Part print with two shaded views. Sizes in mm from the minimum x, y, z corner. Round coordinates to 2 decimals unless told otherwise and drop trailing zeros. Order: outer loops, then holes, each group sorted by start corner. A loop starts at its lowest first (then second) coordinate and runs counter-clockwise, first axis right, second up. Notation, with made-up numbers: (-15, 71.5) - (-2, 71.5) arc R18 cw to (-2, 85.5) - close; hole circle Ø10 at (0, -7.75). An arc over 180 degrees is marked (long way). Answer as CSV lines item,"result". Start each with the question number.
1. Pin check, flat tips, straight feed: pin 1 Ø8 at (x, z) = (75, 8) entering from +Y; pin 2 Ø3 at (x, z) = (85, 27.92) entering from +Y. Stop position of each tip, or through.
2. Pull direction Z, two halves, no side cores. Call the marked faces 1, 2 and 3: released by +Z, released by -Z, zero draft, split by the parting line, or undercut.
3. Band-saw the part on A-A on x = 65. List the corners of the cut face in (y, z) (3 decimals).
4. Band-saw the part on C-C on x = 85. List the corners of the cut face in (y, z) (3 decimals), then the cut area to 3 significant figures.
5. Band-saw the part on B-B on z = 19.5. List the corners of the cut face in (x, y), then the cut area to 3 significant figures.
6. Band-saw the part on D-D on x = 50. List the corners of the cut face in (y, z).
7. Wall check: line 1 along X through (y, z) = (6, 12); line 2 along Z through (x, y) = (15, 5.5); line 3 along Z through (x, y) = (75, 0.25) (3 decimals). Give the ranges that are in metal, low to high. Write a range as [from, to].
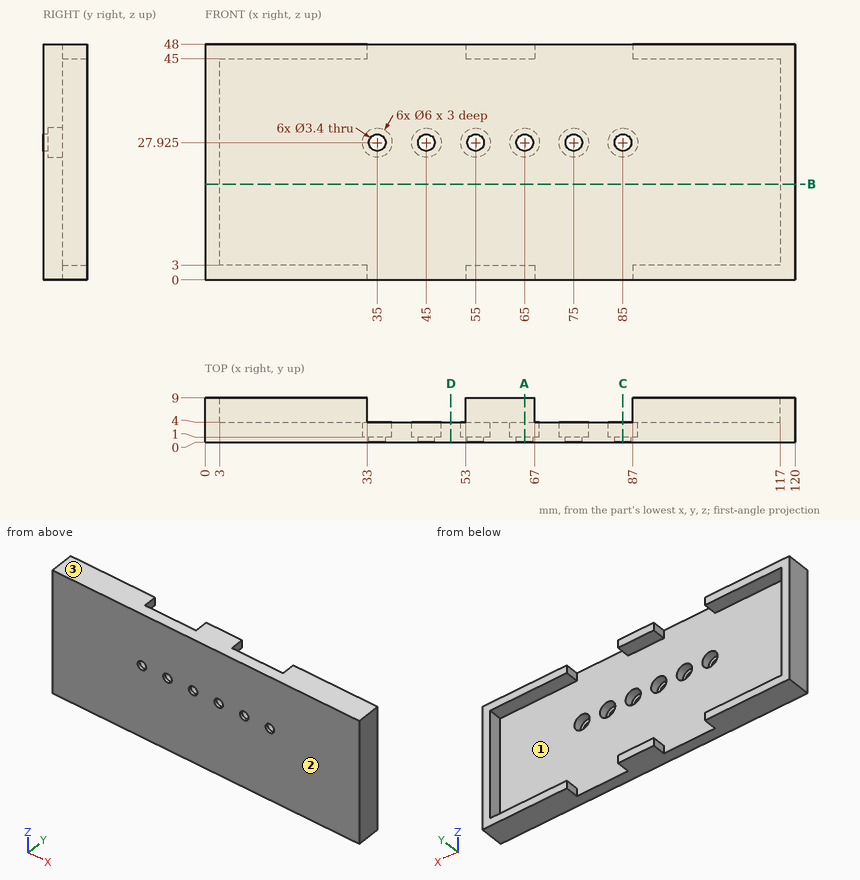
Reply:
1,pin 1,"stops at y = 4"
1,pin 2,"passes through"
2,face 1,"undercut"
2,face 2,"zero draft"
2,face 3,"released by +Z"
3,outline,"(0, 0) - (9, 0) - (9, 3) - (4, 3) - (4, 24.925) - (1, 24.925) - (1, 26.225) - (0, 26.225) - close; (0, 29.625) - (1, 29.625) - (1, 30.925) - (4, 30.925) - (4, 45) - (9, 45) - (9, 48) - (0, 48) - close"
4,outline,"(0, 0) - (4, 0) - (4, 24.925) - (1, 24.925) - (1, 26.225) - (0, 26.225) - close; (0, 29.625) - (1, 29.625) - (1, 30.925) - (4, 30.925) - (4, 48) - (0, 48) - close"
4,area,"171 mm2"
5,outline,"(0, 0) - (120, 0) - (120, 9) - (117, 9) - (117, 4) - (3, 4) - (3, 9) - (0, 9) - close"
5,area,"510 mm2"
6,outline,"(0, 0) - (4, 0) - (4, 48) - (0, 48) - close"
7,line 1,"x = [0, 3], [117, 120]"
7,line 2,"z = [0, 3], [45, 48]"
7,line 3,"z = [0, 26.225], [29.625, 48]"
